Can you work these out from the drawing? Everything is in mm from the part's minimum corner. A direction names the side the tool comes from. Coordinates: 2 decimals unless noted, no trailing zeros. Loops run counter-clockwise (first coordinate to the right, second up) from the corner with the lowest first, then second, coordinate; pieces in that order, holes last.
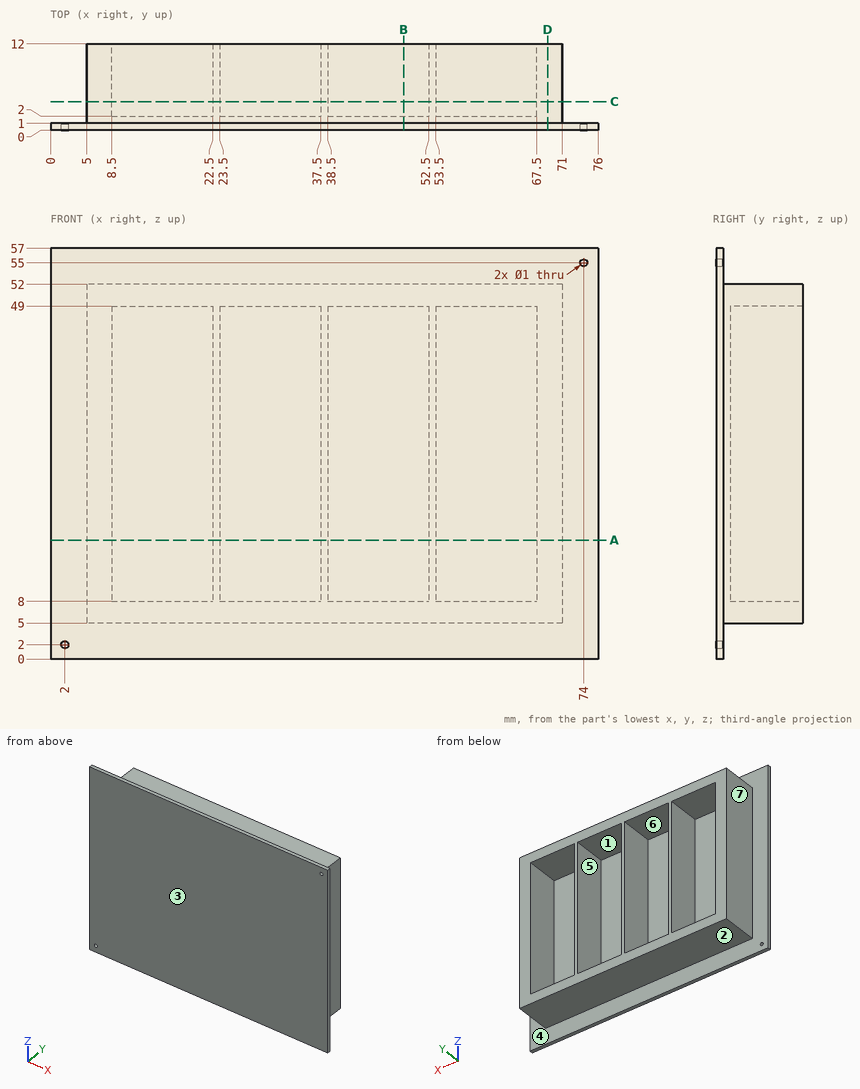
1. I want a section at A-A (z = 16.5). Please give me the cut outline in (x, y), then the cut area to 3 significant figures.
2. I want a section at C-C (y = 4). Please give me the cut outline in (x, z).
3. I want a section at B-B (x = 49). Please give me the cut outline in (y, z).
4. I need wall thicknesses on line 1 along X through (y, z) = (10.75, 11); line 2 along X through (y, z) = (0.7, 55); line 3 along Z through (x, y) = (33.5, 9). Which ranges of each line are inside material? Lowest first, please.
5. I want a section at D-D (x = 69). Please give me the cut outline in (y, z), then the cut area to 3 significant figures.
6. For pin 1 (11 mm diameter, centred on x = 31.5, z = 37.5, fed in from +Y); pin 2 (5 mm diameter, centred on x = 51.5, y = 5, fed in from +Z); pin 3 (5 mm diameter, centred on x = 18.5, y = 7, fed in from -Z), each with a flat end and sliding along its axis, tell me the tip position at first contact or that it passes through.
7. We'd pull the mould along X, two halves only. Please class the marked faces 4, 5, 6 and 7: +X half, -X half, draft (parallel to the pull), parting line (faces both ways), or undercut.
8. On a 3-axis mill with a long thin cutter (end or side, diameter ignored), from which of +Z, -Z, +X, -X, +Y, -Y can I reach the whole of each face in a straight line? I mean the marked faces 1, 2 and 3. Say none if no direction works.
Response values:
1. outline: (0, 0) - (76, 0) - (76, 1) - (71, 1) - (71, 12) - (67.5, 12) - (67.5, 2) - (53.5, 2) - (53.5, 12) - (52.5, 12) - (52.5, 2) - (38.5, 2) - (38.5, 12) - (37.5, 12) - (37.5, 2) - (23.5, 2) - (23.5, 12) - (22.5, 12) - (22.5, 2) - (8.5, 2) - (8.5, 12) - (5, 12) - (5, 1) - (0, 1) - close
1. area: 242 mm2
2. outline: (5, 5) - (71, 5) - (71, 52) - (5, 52) - close; hole (8.5, 8) - (22.5, 8) - (22.5, 49) - (8.5, 49) - close; hole (23.5, 8) - (37.5, 8) - (37.5, 49) - (23.5, 49) - close; hole (38.5, 8) - (52.5, 8) - (52.5, 49) - (38.5, 49) - close; hole (53.5, 8) - (67.5, 8) - (67.5, 49) - (53.5, 49) - close
3. outline: (0, 0) - (1, 0) - (1, 5) - (12, 5) - (12, 8) - (2, 8) - (2, 49) - (12, 49) - (12, 52) - (1, 52) - (1, 57) - (0, 57) - close
4. line 1: x = 5 to 8.5, 22.5 to 23.5, 37.5 to 38.5, 52.5 to 53.5, 67.5 to 71
4. line 2: x = 0 to 73.5, 74.5 to 76
4. line 3: z = 5 to 8, 49 to 52
5. outline: (0, 0) - (1, 0) - (1, 5) - (12, 5) - (12, 52) - (1, 52) - (1, 57) - (0, 57) - close
5. area: 574 mm2
6. pin 1: stops at y = 2
6. pin 2: stops at z = 52
6. pin 3: stops at z = 5
7. face 4: draft
7. face 5: undercut
7. face 6: undercut
7. face 7: -X half
8. face 1: +Y
8. face 2: -Z, +X, -X, +Y
8. face 3: +Z, -Z, +X, -X, -Y
